Verification items for this drawing (mm, ordinates from the low corner). A direction names the side the tool comes from. Coordinates: 2 decimals unless noted, no trailing zeros. Loops run counter-clockwise (first coordinate to the right, second up) from the corner with the lowest first, then second, coordinate; pieces in that order, holes last. Notation, with made-up numbers: M 59,19 L 77,19 A17 cw 77,43 Z; hole C 65,63.25 d10. An arc over 180 degrees is marked long. Return JSON: item names as keys, results as strings.
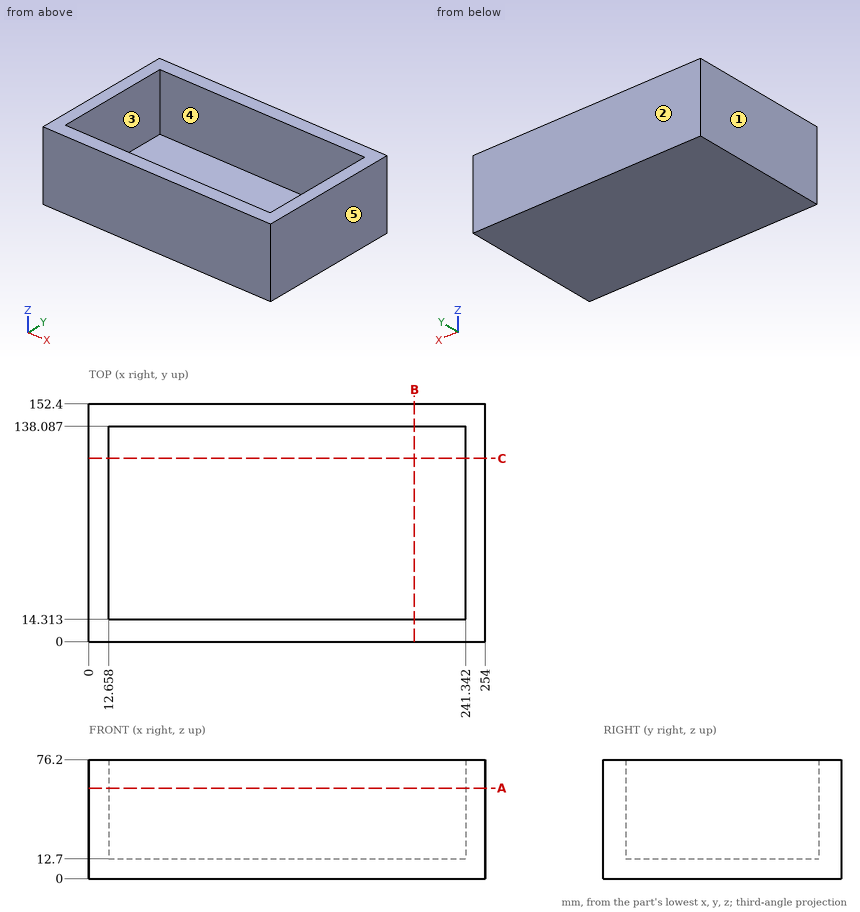
1) Section check B-B on x = 208.5. Record the cut outline in (y, z).
Answers:
{"outline": "M 0,0 L 152.4,0 L 152.4,76.2 L 138.09,76.2 L 138.09,12.7 L 14.31,12.7 L 14.31,76.2 L 0,76.2 Z"}
2) Scan lines: line 1 along X through (y, z) = (101, 68); line 2 along Y through (x, z) = (61, 18.5); line 3 along Z through (x, y) = (118, 30.5). Record each from-to range of solid material in increasing order. Write a range as [from, to].
Answers:
{"line 1": "[0, 12.66], [241.34, 254]", "line 2": "[0, 14.31], [138.09, 152.4]", "line 3": "[0, 12.7]"}
3) Set-up check for the marked faces 4 and 5: record each of +Z, -Z, +X, -X, +Y, -Y from which the full face is reachable in a straight line by a thin tool's end or side.
Answers:
{"face 4": "+Z", "face 5": "+Z, -Z, +X, +Y, -Y"}
4) Section check A-A on z = 58. Record the cut outline in (x, y).
Answers:
{"outline": "M 0,0 L 254,0 L 254,152.4 L 0,152.4 Z; hole M 12.66,14.31 L 241.34,14.31 L 241.34,138.09 L 12.66,138.09 Z"}
5) Draft check along Y on the marked faces 1, 2 and 3. Enter one of: +Y half, -Y half, draft (parallel to the pull), parting line (faces both ways), or undercut.
Answers:
{"face 1": "draft", "face 2": "+Y half", "face 3": "undercut"}
6) Section check C-C on y = 117.5. Record the cut outline in (x, z), then the cut area to 3 significant figures.
Answers:
{"outline": "M 0,0 L 254,0 L 254,76.2 L 241.34,76.2 L 241.34,12.7 L 12.66,12.7 L 12.66,76.2 L 0,76.2 Z", "area": "4,830 mm²"}
7) Go/stop test with a flat-tipped pin: pin 1 Ø3 at (x, y) = (86, 123) entering from +Z. Record where the tip stops, or that it passes through.
Answers:
{"pin 1": "z = 12.7"}
